from build123d import *

# Parameters (mm, degrees)
SKETCH2_R           = 0.500109693
BOSS_EXTRUDE1_DEPTH = 5
BOSS_EXTRUDE2_DEPTH = 1


with BuildPart() as part:
    # Sketch2 → Boss-Extrude1 (new body)
    with BuildSketch(Plane(origin=(0, 0, 0), x_dir=(1, 0, 0), z_dir=(0, 0, -1))):
        with BuildLine():
            Line((29.97295835, 6.642737104), (28.862437793, 5.215722686))
            Line((28.862437793, 5.215722686), (29.97295835, 3.953817374))
            add(Edge.make_bspline(
                [(5.565346412, 3.953817374), (17.919076804, -3.939717318), (29.97295835, 3.953817374)],
                knots=[0, 0, 0, 1, 1, 1], degree=2))
            Line((5.565346412, 3.953817374), (0, 0.570103483))
            Line((0, 0.570103483), (2.65645961, 5.215722686))
            Line((2.65645961, 5.215722686), (0, 9.556126627))
            Line((0, 9.556126627), (5.565346412, 6.285726684))
            add(Edge.make_bspline(
                [(5.565346412, 6.285726684), (12.037313538, 11.217277608), (22.14175538, 12.07873787), (29.97295835, 6.642737104)],
                knots=[0, 0, 0, 0, 1, 1, 1, 1], degree=3))
        make_face()
        with Locations(Location((26.5225963, 6.780666166, 0), (0, 0, 180))):
            Circle(SKETCH2_R, mode=Mode.SUBTRACT)
    extrude(amount=-BOSS_EXTRUDE1_DEPTH)

    # Sketch6 → Boss-Extrude2 (add)
    with BuildSketch(Plane(origin=(0, 0, 5), x_dir=(-1, 0, 0), z_dir=(0, 0, 1))):
        with BuildLine():
            Line((-15.759449442, 1.418953032), (-16.07584813, 3.995005952))
            add(Edge.make_bspline(
                [(-16.07584813, 3.995005952), (-15.458880746, 4.062710088), (-14.740919917, 4.238390229), (-14.650433604, 5.193040536)],
                knots=[0, 0, 0, 0, 1, 1, 1, 1], degree=3))
            add(Edge.make_bspline(
                [(-14.650433604, 5.193040536), (-14.619231687, 5.862120963), (-15.169780731, 6.414980417), (-16.232102989, 6.432436177)],
                knots=[0, 0, 0, 0, 1, 1, 1, 1], degree=3))
            add(Edge.make_bspline(
                [(-16.232102989, 6.432436177), (-17.005188221, 6.511841439), (-17.780119933, 5.869895845), (-17.317691742, 4.369140076)],
                knots=[0, 0, 0, 0, 1, 1, 1, 1], degree=3))
            Line((-17.317691742, 4.369140076), (-19.0853994, 4.482638032))
            add(Edge.make_bspline(
                [(-19.0853994, 4.482638032), (-19.056118502, 4.997195312), (-19.258203254, 6.439044313), (-20.66941937, 5.911436499)],
                knots=[0, 0, 0, 0, 1, 1, 1, 1], degree=3))
            add(Edge.make_bspline(
                [(-20.66941937, 5.911436499), (-21.486344473, 5.457892375), (-21.162251573, 3.883318696), (-19.884325096, 3.995005952)],
                knots=[0, 0, 0, 0, 1, 1, 1, 1], degree=3))
            Line((-19.884325096, 3.995005952), (-20.327479071, 1.52976102))
            add(Edge.make_bspline(
                [(-22.787674533, 5.404891959), (-22.963836678, 3.337144225), (-21.949807027, 1.978010395), (-20.327479071, 1.52976102)],
                knots=[0, 0, 0, 0, 1, 1, 1, 1], degree=3))
            add(Edge.make_bspline(
                [(-18.474874193, 7.338129926), (-19.24932143, 9.101790183), (-22.509278972, 9.429289769), (-22.787674533, 5.404891959)],
                knots=[0, 0, 0, 0, 1, 1, 1, 1], degree=3))
            add(Edge.make_bspline(
                [(-16.07584813, 9.06636742), (-17.73342296, 9.193466544), (-18.474874193, 7.338129926)],
                knots=[0, 0, 0, 1, 1, 1], degree=2))
            add(Edge.make_bspline(
                [(-13.123671188, 5.404891959), (-13.173598197, 6.971888977), (-14.244410718, 9.017312988), (-16.07584813, 9.06636742)],
                knots=[0, 0, 0, 0, 1, 1, 1, 1], degree=3))
            add(Edge.make_bspline(
                [(-15.759449442, 1.418953032), (-13.321402819, 1.889445376), (-13.053480895, 4.428709713), (-13.123671188, 5.404891959)],
                knots=[0, 0, 0, 0, 1, 1, 1, 1], degree=3))
        make_face()
    extrude(amount=BOSS_EXTRUDE2_DEPTH)


solid = part.part
Verification items for the finished model (mm, model axes). A direction names the side the tool comes from. Round coordinates to 2 decimals unless told otherwise and drop trailing zeros. Use a Markdown table: item, result. Add a question column.
1. Thickness scan on probe 1 along Z at (x, y) = (15.25, -0.75); probe 2 along X at (y, z) = (-2.5, 2); probe 3 along X at (y, z) = (-1.75, 2.5). Record the ranges inside material, lowest first. Write a range as [from, to].
2. Access from +Z, -Z, +X, -X, +Y, -Y to the whole of each face (thin tool, end or side, straight path). Record for faces 1 (the face through (2.822, -2.286, 2.465)), 2 (the face through (1.31, -2.86, 2.46)), 3 (the face through (29.425, -5.939, 2.465)), 4 (the face through (20.1, -2.8, 5.5)), 5 (the face through (2.744, -7.944, 2.465)).
3. Gauge pin test, flat end, axial feed: pin 1 (0.8 mm diameter, centred on x = 26.52, y = -6.78, fed in from +Z). Record the tip position at first contact, or that the pin passes through.
Checks:
| question | item | result |
|---|---|---|
| 1 | probe 1 | z = [0, 5] |
| 1 | probe 2 | x = [1.1, 3.17], [8.1, 27.5] |
| 1 | probe 3 | x = [0.67, 1.94], [9.7, 25.92] |
| 2 | face 1 | +Z, -Z, +Y |
| 2 | face 2 | +Z, -Z, -X |
| 2 | face 3 | +Z, -Z, +X |
| 2 | face 4 | +Z, +Y |
| 2 | face 5 | +Z, -Z, -Y |
| 3 | pin 1 | passes through |
